Check sheet for the modelled part. Datum: model origin and axes. Units: mm. A direction names the side the tool comes from. Round coordinates to 2 decimals unless told otherwise and drop trailing zeros. Order: outer loops, then holes, each group sorted by start corner. A loop starts at its lowest first (then second) coordinate and runs counter-clockwise, first axis right, second up. Notation, with made-up numbers: (32.25, 30.5) -> (76.25, 30.5) arc R19 ccw to (76.25, 35.5) -> close; hole circle Ø4 at (21, 25). An arc over 180 degrees is marked (long way). Answer in a Markdown table with one row per item. Add a question column.
1. Depth check by flat-ended pin: P1, Ø4, axis at y = 3.5, z = 26.5, coming from the -X side; P2, Ø1, axis at x = 12.5, y = 1.5, coming from the -Z side; P3, Ø1.6, axis at x = 12.5, y = 1, coming from the +Z side. Enter the tip coordinate at first touch or a pass-through.
2. Sectioned sample at A-A, the plane z = 51.5. Record the boundary of the cut face in (x, y), then the cut area to 3 significant figures.
3. Material ranges on L1, parallel to Y at x = 9.5, z = 30.5; L2, parallel to X at y = 5, z = 9; L3, parallel to Y at x = 3, z = 37.5, recorded low to high. Write a range as from..to.
4. Sectioned sample at B-B, the plane x = 10.75. Record the boundary of the cut face in (y, z), then the cut area to 3 significant figures.
5. Access from +Z, -Z, +X, -X, +Y, -Y to the whole of each face (thin tool, end or side, straight path). Record for faces 4 (the flat face through (11.7, 1, 20)), 5 (the flat face through (-4.7, 1, 40)), 6 (the flat face through (2.966, 4, 30)), 7 (the flat face through (11.419, 1, 50)), 8 (the cylindrical face through (-5.85, 0.81, 9.86)).
6. Draft check along Z on faces 1 (the flat face through (2, 1, 60)), 2 (the flat face through (-4.391, 1, 30)), 3 (the flat face through (-3, 0, 30)). Enter one of: +Z half, -Z half, draft (parallel to the pull), parting line (faces both ways), or undercut.
7. Sectioned sample at C-C, the plane x = 6.5. Record the boundary of the cut face in (y, z).
```python
from build123d import *

# Parameters (mm, degrees)
SKETCH1_W           = 20
SKETCH1_H           = 2
BOSS_EXTRUDE1_DEPTH = 60
CUT_EXTRUDE2_DEPTH  = 70
SKETCH5_R           = 0.5
CUT_EXTRUDE3_DEPTH  = 70
SKETCH6_W           = 2
SKETCH6_H           = 20
CUT_EXTRUDE4_DEPTH  = 70
SKETCH7_W           = 2
SKETCH7_H           = 5
BOSS_EXTRUDE2_DEPTH = 60
SKETCH9_W           = 8
SKETCH9_H           = 60
CUT_EXTRUDE5_DEPTH  = 1
BOSS_EXTRUDE3_DEPTH = 60


with BuildPart() as part:
    # Sketch1 → Boss-Extrude1 (new body)
    with BuildSketch(Plane.XY):
        with Locations((3.513513514, 1)):
            Rectangle(SKETCH1_W, SKETCH1_H)
    extrude(amount=BOSS_EXTRUDE1_DEPTH)

    # Sketch4 → Cut-Extrude2 (cut)
    with BuildSketch(Plane(origin=(0, 0, 0), x_dir=(-1, 0, 0), z_dir=(0, 0, -1))):
        with BuildLine():
            Line((-13.513513514, 2), (-12.513513514, 2))
            ThreePointArc((-12.513513514, 2), (-13.417253411, 0.949937849), (-12.413513514, -0.004987562))
            Line((-12.413513514, -0.004987562), (-13.513513514, -0.004987562))
            Line((-13.513513514, -0.004987562), (-13.513513514, 2))
        make_face()
        with BuildLine():
            Line((6.486486486, 2), (5.486486486, 2))
            ThreePointArc((5.486486486, 2), (6.390226384, 0.949937849), (5.386486486, -0.004987562))
            Line((5.386486486, -0.004987562), (6.486486486, -0.004987562))
            Line((6.486486486, -0.004987562), (6.486486486, 2))
        make_face()
    extrude(amount=-CUT_EXTRUDE2_DEPTH, mode=Mode.SUBTRACT)

    # Sketch5 → Cut-Extrude3 (cut)
    with BuildSketch(Plane(origin=(0, 0, 0), x_dir=(-1, 0, 0), z_dir=(0, 0, -1))):
        with Locations((-12.413513514, 1)):
            Circle(SKETCH5_R)
        with Locations((5.386486486, 1)):
            Circle(SKETCH5_R)
    extrude(amount=-CUT_EXTRUDE3_DEPTH, mode=Mode.SUBTRACT)

    # Sketch6 → Cut-Extrude4 (cut)
    with BuildSketch(Plane(origin=(0, 2, 0), x_dir=(1, 0, 0), z_dir=(0, 1, 0))):
        with Locations((-5.391474049, -30)):
            Rectangle(SKETCH6_W, SKETCH6_H)
        with Locations((12.418501076, -10)):
            Rectangle(SKETCH6_W, SKETCH6_H)
        with Locations((12.418501076, -50)):
            Rectangle(SKETCH6_W, SKETCH6_H)
    extrude(amount=-CUT_EXTRUDE4_DEPTH, mode=Mode.SUBTRACT)

    # Sketch7 → Boss-Extrude2 (add)
    with BuildSketch(Plane(origin=(0, 0, 0), x_dir=(-1, 0, 0), z_dir=(0, 0, -1))):
        with Locations((-3.966007295, 4.5)):
            Rectangle(SKETCH7_W, SKETCH7_H)
    extrude(amount=-BOSS_EXTRUDE2_DEPTH)

    # Sketch9 → Cut-Extrude5 (cut)
    with BuildSketch(Plane(origin=(0, 0, 0), x_dir=(-1, 0, 0), z_dir=(0, -1, 0))):
        with Locations((-3.418501076, -30)):
            Rectangle(SKETCH9_W, SKETCH9_H)
    extrude(amount=-CUT_EXTRUDE5_DEPTH, mode=Mode.SUBTRACT)

    # Sketch12 → Boss-Extrude3 (add)
    with BuildSketch(Plane(origin=(0, 0, 0), x_dir=(-1, 0, 0), z_dir=(0, 0, -1))):
        with BuildLine():
            Line((-7.418501076, 1), (0.581498924, 1))
            Line((0.581498924, 1), (0.581498924, 0))
            ThreePointArc((0.581498924, 0), (-3.418501076, 0.188654004), (-7.418501076, 0))
            Line((-7.418501076, 0), (-7.418501076, 1))
        make_face()
    extrude(amount=-BOSS_EXTRUDE3_DEPTH)


solid = part.part
```
Answer key:
| question | item | result |
|---|---|---|
| 1 | P1 | stops at x = -4.39 |
| 1 | P2 | stops at z = 20 |
| 1 | P3 | stops at z = 40 |
| 2 | outline | (-5.49, 0) -> (-0.58, 0) arc R42.5 cw to (7.42, 0) -> (11.42, 0) -> (11.42, 2) -> (4.97, 2) -> (4.97, 7) -> (2.97, 7) -> (2.97, 2) -> (-5.49, 2) arc R1 ccw to start; hole circle Ø1 at (-5.39, 1) |
| 2 | area | 43.4 mm² |
| 3 | L1 | y = 0..2 |
| 3 | L2 | x = 2.97..4.97 |
| 3 | L3 | y = 0.19..7 |
| 4 | outline | (0, 0) -> (2, 0) -> (2, 60) -> (0, 60) -> close |
| 4 | area | 120 mm² |
| 5 | face 4 | -Z, +X, +Y, -Y |
| 5 | face 5 | -X, +Y, -Y |
| 5 | face 6 | +Z, -Z, -X, +Y |
| 5 | face 7 | +Z, +X, +Y, -Y |
| 5 | face 8 | +Z, -Z |
| 6 | face 1 | +Z half |
| 6 | face 2 | undercut |
| 6 | face 3 | draft |
| 7 | outline | (0.08, 0) -> (2, 0) -> (2, 60) -> (0.08, 60) -> close |
